Can you work these out from the model? Positions are in its coordinate system, mm. Coordinates: 2 decimals unless noted, no trailing zeros. Order: outer loops, then holes, each group sorted by start corner. A loop starts at its lowest first (then second) coordinate and runs counter-clockwise, first axis right, second up. Notation, with made-up numbers: M 12,63.5 L 66,63.5 A10 cw 66,78.5 Z; hole C -13,89.5 d2. An arc over 180 degrees is marked long. Answer as a JSON object with one key per item and string values.
Autodesk Inventor part; units mm, degrees
ref_plane "YZ Plane" through (0, 0, 0) normal (1, 0, 0) x (0, 1, 0)
ref_plane "XZ Plane" through (0, 0, 0) normal (0, 1, 0) x (-1, 0, 0)
ref_plane "XY Plane" through (0, 0, 0) normal (0, 0, 1) x (1, 0, 0)
sketch "Sketch1" plane through (0, 0, 0) normal (0, 1, 0) x (-1, 0, 0)
  line L0 (-10, 5) -> (10, 5)
  line L1 (10, 5) -> (10, -5)
  line L2 (10, -5) -> (-10, -5)
  line L3 (-10, -5) -> (-10, 5)
  line L4 (-10, 5) -> (10, -5) construction
  line L5 (10, 5) -> (-10, -5) construction
  point P0 (0, 0)
  dimension "d0" = 20
  dimension "d1" = 10
extrude "Extrusion1" add sketch "Sketch1" along normal blind 300
sketch "Sketch2" plane through (0, 300, 0) normal (0, 1, 0) x (1, 0, 0)
  line L0 (0, 0) -> (0, 3.3139) construction
  line L1 (10, 5) -> (-10, 5)
  circle A0 centre (-5, 0) radius 2
  circle A1 centre (5, 0) radius 2
  line L2 (0, 0) -> (-5, 0)
  line L3 (0, 0) -> (5, 0)
  dimension "d4" = 4
  dimension "d7" = 5
  dimension "d8" = 5
extrude "Extrusion2" cut sketch "Sketch2" against normal blind 300
sketch "Sketch3" plane through (-10, 0, -5) normal (-1, 0, 0) x (0, 0, 1)
  line L0 (0, 300) -> (10, 300)
  line L1 (5, 300) -> (5, 295) construction
  line L2 (5, 295) -> (5, 285) construction
  circle A0 centre (5, 295) radius 1.6538
  circle A1 centre (5, 285) radius 2
  point P0 (5, 0)
  dimension "d9" = 5
  dimension "d10" = 10
  dimension "d11" = 4
extrude "Extrusion3" cut sketch "Sketch3" against normal blind 32.225
properties part number "spine"
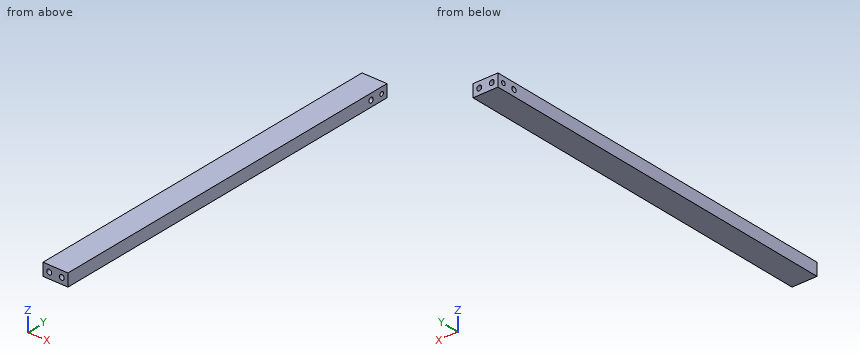
Item 1: I want a section at B-B, the plane z = 0. Give the number of separate pieces and of enclosed holes in the cut face, plus the area to 3 significant figures.
Answers follow:
{"separate pieces": "9", "enclosed holes": "0", "area": "3,510 mm^2"}
Item 2: I'm going to push flat-ended pins straight in: pin 1 (3 mm diameter, centred on x = 5, z = -1.5, fed in from +Y); pin 2 (3 mm diameter, centred on y = 285, z = 0, fed in from -X). Where does each tip first touch, or does it pass through?
Answers follow:
{"pin 1": "stops at y = 300", "pin 2": "passes through"}
Item 3: Please list where these lines run through material, in increasing order: line 1 (X direction, y = 269.5, z = 0.25); line 2 (Y direction, x = 7.1, z = 0); line 3 (X direction, y = 89, z = 1.75).
Answers follow:
{"line 1": "x = -10 to -6.98, -3.02 to 3.02, 6.98 to 10", "line 2": "y = 0 to 283, 287 to 293.35, 296.65 to 300", "line 3": "x = -10 to -5.97, -4.03 to 4.03, 5.97 to 10"}
Item 4: I want a section at A-A, the plane y = 245. Write out the boundary of the cut face in (x, z), plus the area to 3 significant figures.
Answers follow:
{"outline": "M -10,-5 L 10,-5 L 10,5 L -10,5 Z; hole C -5,0 d4; hole C 5,0 d4", "area": "175 mm^2"}
